Could you check a few things on this model? Use its own coordinates, in mm. Face numbers are marked on the shaded views. A direction names the side the tool comes from. Give positions to 0.01 mm unless a question says otherwise; leave off trailing zeros. Write each loop counter-clockwise with the first axis right and the second up, starting at its lowest first coordinate (ties: lowest second). Pieces come first, ordered by that corner, then holes. Notation, with made-up numbers: (11, 27.25) -> (27, 27.25) arc R26 cw to (27, 63.25) -> close; hole circle Ø2 at (44, -28). An arc over 180 degrees is marked (long way). One line per question, with ' | ' between items.
from build123d import *

# Parameters (mm, degrees)
F0_R      = 12.573
F1_DEPTH  = 31.75
F3_W      = 12.7
F3_H      = 20.32
F4_DEPTH  = 6.986
F6_W      = 6.35
F6_H      = 20.066
F7_DEPTH  = 10.161
F8_W      = 8.89
F8_H      = 17.78
F9_DEPTH  = 12.574
F10_R     = 6.35
F11_DEPTH = 31.751
F12_R     = 9.525
F13_DEPTH = 25.4


with BuildPart() as f1:
    # F0 (on Top) → F1 (new body)
    with BuildSketch(Plane.XY):
        Circle(F0_R)
    extrude(amount=F1_DEPTH)

    # F3 (on offset) → F4 (cut, through all)
    with BuildSketch(Plane.YZ.offset(5.588)):
        with Locations((0, 15.24)):
            Rectangle(F3_W, F3_H)
    extrude(amount=F4_DEPTH, mode=Mode.SUBTRACT)

    # F6 (on offset) → F7 (cut, through all)
    with BuildSketch(Plane.XZ.offset(-2.413)):
        with Locations((0, 13.208)):
            Rectangle(F6_W, F6_H)
    extrude(amount=-F7_DEPTH, mode=Mode.SUBTRACT)

    # F8 (on Front) → F9 (cut, through all)
    with BuildSketch(Plane.XZ):
        with Locations((0, 15.24)):
            Rectangle(F8_W, F8_H)
    extrude(amount=F9_DEPTH, mode=Mode.SUBTRACT)

    # F10 (on Top) → F11 (cut, through all)
    with BuildSketch(Plane.XY):
        Circle(F10_R)
    extrude(amount=F11_DEPTH, mode=Mode.SUBTRACT)

    # F12 (on face) → F13 (cut)
    with BuildSketch(Plane(origin=(0, 0, 0), x_dir=(1, 0, 0), z_dir=(0, 0, -1))):
        Circle(F12_R)
    extrude(amount=-F13_DEPTH, mode=Mode.SUBTRACT)


solid = f1.part
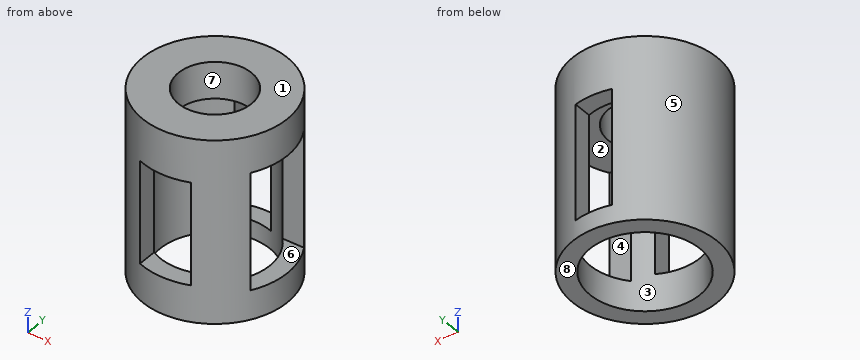
Q1. On a 3-axis mill with a long thin cutter (end or side, diameter ignored), from which of +Z, -Z, +X, -X, +Y, -Y can I reach the whole of each face in a straight line? I mean the marked faces 1, 2, 3, 4 and 5. Say none if no direction works.
Answer below:
face 1: +Z, +X, -X, +Y, -Y | face 2: none | face 3: -Z | face 4: +X | face 5: +Z, -Z
Q2. Imagine slicing it at B-B on z = 14.5. Please give me the cut outline in (x, y) (3 decimals).
Answer below:
outline: (-4.445, -11.761) -> (-4.445, -8.424) arc R9.525 cw to (-3.175, 8.98) -> (-3.175, 12.166) arc R12.573 ccw to start; (3.175, 8.98) arc R9.525 cw to (7.1, 6.35) -> (10.852, 6.35) arc R12.573 ccw to (3.175, 12.166) -> close; (4.445, -11.761) arc R12.573 ccw to (10.852, -6.35) -> (7.1, -6.35) arc R9.525 cw to (4.445, -8.424) -> close
Q3. Imagine slicing it at D-D on y = -6.75. Please give me the cut outline in (x, z), and give its area (3 significant figures).
Answer below:
outline: (-10.61, 0) -> (-6.72, 0) -> (-6.72, 25.4) -> (6.72, 25.4) -> (6.72, 0) -> (10.61, 0) -> (10.61, 31.75) -> (-10.61, 31.75) -> close | area: 332 mm^2
Q4. Imagine slicing it at C-C on y = 0. Please give me the cut outline in (x, z) (3 decimals).
Answer below:
outline: (-12.573, 0) -> (-9.525, 0) -> (-9.525, 25.4) -> (-6.35, 25.4) -> (-6.35, 31.75) -> (-12.573, 31.75) -> close; (6.35, 25.4) -> (12.573, 25.4) -> (12.573, 31.75) -> (6.35, 31.75) -> close; (9.525, 0) -> (12.573, 0) -> (12.573, 5.08) -> (9.525, 5.08) -> close
Q5. If I drill on line 1 along Z through (x, y) = (-1.25, 9.5) (3 decimals); line 2 along Y through (x, z) = (0, 30.25); line 3 along Z through (x, y) = (0.75, 8.25), over which ranges is the centre line in solid material (lowest first)?
Answer below:
line 1: z = 0 to 3.175, 23.241 to 31.75 | line 2: y = -12.57 to -6.35, 6.35 to 12.57 | line 3: z = 25.4 to 31.75
Q6. Will these pins go through, and if not, where does the flat tip stop? pin 1 (1.5 mm diameter, centred on x = -6, y = 10, fed in from -Z); pin 2 (1 mm diameter, centred on y = 10, z = 13.5, fed in from -X); pin 3 (1.7 mm diameter, centred on y = -11, z = 18, fed in from +X); pin 4 (3.5 mm diameter, centred on y = -9.5, z = 16.5, fed in from -X).
Answer below:
pin 1: stops at z = 0 | pin 2: stops at x = -8.24 | pin 3: stops at x = 7.42 | pin 4: stops at x = -9.9
Q7. Imagine slicing it at A-A on x = 0. Please give me the cut outline in (y, z) (3 decimals).
Answer below:
outline: (-12.573, 0) -> (-9.525, 0) -> (-9.525, 6.35) -> (-12.573, 6.35) -> close; (-12.573, 24.13) -> (-9.525, 24.13) -> (-9.525, 25.4) -> (-6.35, 25.4) -> (-6.35, 31.75) -> (-12.573, 31.75) -> close; (6.35, 25.4) -> (9.525, 25.4) -> (9.525, 23.241) -> (12.573, 23.241) -> (12.573, 31.75) -> (6.35, 31.75) -> close; (9.525, 0) -> (12.573, 0) -> (12.573, 3.175) -> (9.525, 3.175) -> close
Q8. If we mould it in two halves opening along Z, with no side actions, what happens to the marked faces 6, 7 and 8? For each: +Z half, -Z half, draft (parallel to the pull), parting line (faces both ways), or undercut.
Answer below:
face 6: undercut | face 7: draft | face 8: -Z half
